Here's how the part is built. I have some questions about the finished solid (model axes, mm). A direction names the side the tool comes from. Round coordinates to 2 decimals unless told otherwise and drop trailing zeros. Order: outer loops, then holes, each group sorted by start corner. A loop starts at its lowest first (then second) coordinate and runs counter-clockwise, first axis right, second up.
```python
from build123d import *

# Parameters (mm, degrees)
BOSS_EXTRUDE1_DEPTH = 5.842
SKETCH2_W           = 0.854807692
SKETCH2_H           = 9.525
CUT_EXTRUDE1_DEPTH  = 3.175


with BuildPart() as part:
    # Sketch1 → Boss-Extrude1 (new body)
    with BuildSketch(Plane.XY):
        Polygon((56.642, -22.225), (-56.642, -22.225), (-56.642, -19.05), (-62.484, -19.05), (-62.484, -6.35), (-56.642, -6.35), (-56.642, 6.35), (-62.484, 6.35), (-62.484, 19.05), (-56.642, 19.05), (-56.642, 22.225), (56.642, 22.225), (56.642, 19.05), (62.484, 19.05), (62.484, 6.35), (56.642, 6.35), (56.642, -6.35), (62.484, -6.35), (62.484, -19.05), (56.642, -19.05), align=None)
    extrude(amount=BOSS_EXTRUDE1_DEPTH)

    # Sketch2 → Cut-Extrude1 (cut)
    with BuildSketch(Plane.XY.offset(5.842)):
        Polygon((-14.104326923, 4.772358215), (-14.104326923, 5.749281292), (-9.097596154, 5.749281292), (-9.097596154, 4.772358215), (-11.173557692, 4.772358215), (-11.173557692, -3.775718708), (-12.028365385, -3.775718708), (-12.028365385, 4.772358215), align=None)
        with Locations((-7.204807692, 0.986781292)):
            Rectangle(SKETCH2_W, SKETCH2_H)
        Polygon((-4.335096154, -3.775718708), (-4.335096154, 5.749281292), (-4.155739183, 5.749281292), (2.137019231, -1.747458491), (2.137019231, 5.749281292), (2.991826923, 5.749281292), (2.991826923, -3.775718708), (2.797205529, -3.775718708), (-3.480288462, 3.7038486), (-3.480288462, -3.775718708), align=None)
        Polygon((9.341826923, 5.749281292), (13.737980769, -3.775718708), (12.808759014, -3.775718708), (11.400615986, -0.722834092), (7.082692308, -0.722834092), (5.634480168, -3.775718708), (4.701442308, -3.775718708), (9.219711538, 5.749281292), align=None)
        Polygon((9.271228966, 3.892745835), (7.546349159, 0.254088984), (10.950315505, 0.254088984), align=None, mode=Mode.SUBTRACT)
    extrude(amount=-CUT_EXTRUDE1_DEPTH, mode=Mode.SUBTRACT)


solid = part.part
```
1. On a 3-axis mill with a long thin cutter (end or side, diameter ignored), from which of +Z, -Z, +X, -X, +Y, -Y can I reach the whole of each face in a straight line? I mean faces 1 (the flat face through (8.42, 2.1, 4.28)), 2 (the flat face through (-56.642, -21, 3)), 3 (the flat face through (-60, 6.35, 3)). Say none if no direction works.
Evaluation:
face 1: +Z
face 2: +Z, -Z, -X, -Y
face 3: +Z, -Z, -X
2. I need wall thicknesses on probe 1 along Y at (x, z) = (-10, 3.9) (3 decimals); probe 2 along X at (y, z) = (4, 2.8); probe 3 along X at (y, z) = (-3.5, 1.8). Which ranges of each line are inside material? Lowest first, please.
Evaluation:
probe 1: y = -22.225 to 4.772, 5.749 to 22.225
probe 2: x = -56.64 to -12.03, -11.17 to -7.63, -6.78 to -4.34, -2.69 to 2.14, 2.99 to 8.39, 10.15 to 56.64
probe 3: x = -56.64 to 56.64
3. If we section it at B-B, the plane y = -5: Write out the boundary of the cut face in (x, z).
Evaluation:
outline: (-56.64, 0) - (56.64, 0) - (56.64, 5.84) - (-56.64, 5.84) - close
4. I'm going to push flat-ended pins straight in: P1, Ø1, axis at y = 0, z = 3.5, coming from the -X side; P2, Ø1.6, axis at y = 0.5, z = 4, coming from the +X side; P3, Ø3, axis at x = 58.5, z = 3, coming from the +Y side. Where does each tip first touch, or does it pass through?
Evaluation:
P1: stops at x = -56.64
P2: stops at x = 56.64
P3: stops at y = 19.05
5. If we mould it in two halves opening along Y, with no side actions, what happens to faces 4 (the flat face through (-10, 4.772, 4)), 5 (the flat face through (-1.05, 2.05, 4.28)), 6 (the flat face through (56.642, -21, 3)), 7 (the flat face through (-1, 22.225, 3))? For each: released by +Y, released by -Y, zero draft, split by the parting line, or undercut.
Evaluation:
face 4: undercut
face 5: undercut
face 6: zero draft
face 7: released by +Y
6. If we section it at A-A, the plane z = 4.3: State how many separate pieces and enclosed holes the cut face has, and give its area (3 significant figures).
Evaluation:
separate pieces: 2
enclosed holes: 4
area: 5,270 mm2
